The figure shows three views and two pictorial views of one solid part (mm, origin at its lowest corner). Answer the questions. A direction names the side the tool comes from. Round coordinates to 2 decimals unless told otherwise and drop trailing zeros. Order: outer loops, then holes, each group sorted by start corner. A loop starts at its lowest first (then second) coordinate and runs counter-clockwise, first axis right, second up. Notation, with made-up numbers: (-4, 82.25) - (15, 82.25) arc R9 ccw to (15, 92.25) - close; hole circle Ø4 at (32, 39). An arc over 180 degrees is marked (long way). Use CSV: the item, a comma, the result in double quotes.
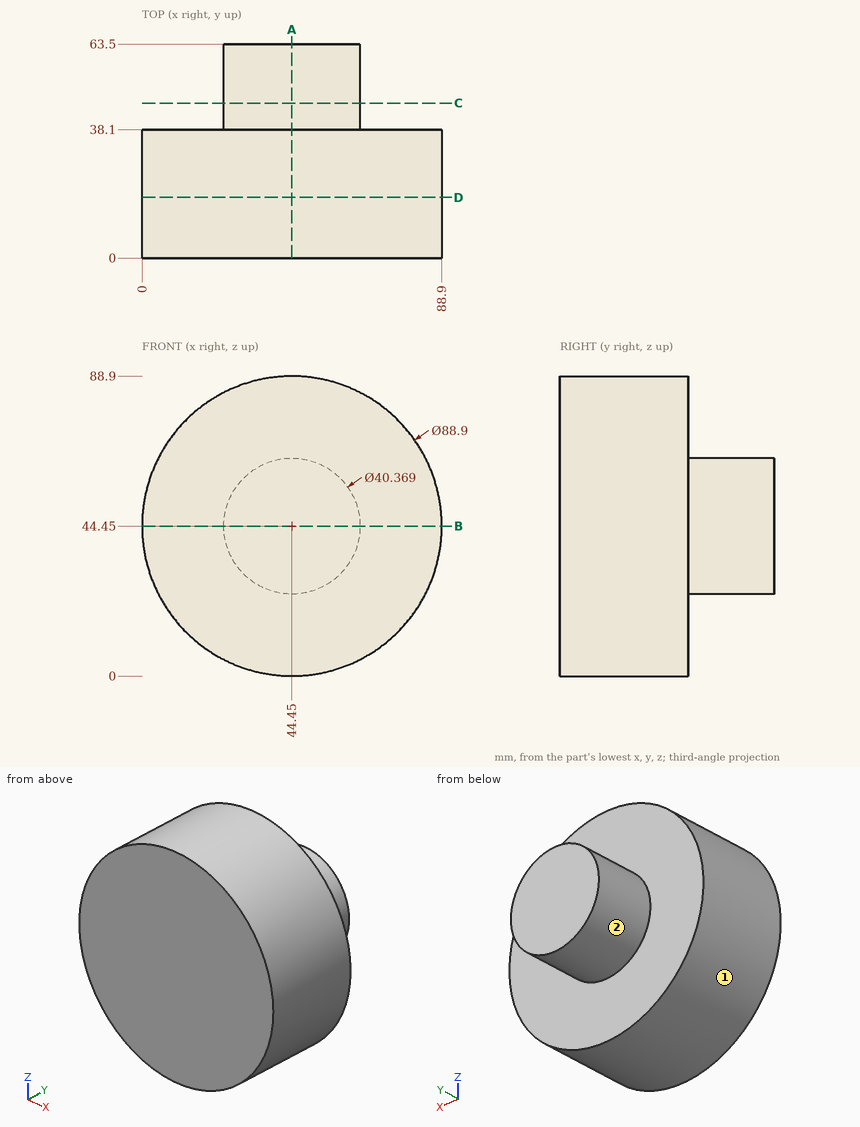
(1) Find section C-C (y = 46). Determine the outline of the cut face in (x, z).
Findings below:
outline,"circle Ø40.37 at (44.45, 44.45)"
(2) Each of these flat-tipped pins is pushed along its axis until it touches: pin 1 (8 mm diameter, centred on x = 70.5, y = 18, fed in from +Z); pin 2 (6 mm diameter, centred on x = 76, z = 49, fed in from +Y); pin 3 (8 mm diameter, centred on y = 10, z = 72, fed in from -X). Where does it stop, or does it pass through?
Findings below:
pin 1,"stops at z = 83.05"
pin 2,"stops at y = 38.1"
pin 3,"stops at x = 6.75"
(3) Find section A-A (x = 44.45). Determine the outline of the cut face in (y, z), and give its area (3 significant figures).
Findings below:
outline,"(0, 0) - (38.1, 0) - (38.1, 24.27) - (63.5, 24.27) - (63.5, 64.63) - (38.1, 64.63) - (38.1, 88.9) - (0, 88.9) - close"
area,"4,410 mm²"
(4) Find section D-D (y = 18). Determine the outline of the cut face in (x, z).
Findings below:
outline,"circle Ø88.9 at (44.45, 44.45)"
(5) Find section B-B (z = 44.45). Determine the outline of the cut face in (x, y).
Findings below:
outline,"(0, 0) - (88.9, 0) - (88.9, 38.1) - (64.63, 38.1) - (64.63, 63.5) - (24.27, 63.5) - (24.27, 38.1) - (0, 38.1) - close"
(6) For the marked faces 1 and 2, determine the directions among +Z, -Z, +X, -X, +Y, -Y from which every point of the face is accessible in a straight line to the end or side of a thin tool.
Findings below:
face 1,"+Y, -Y"
face 2,"+Y"
(7) Find the intervals of material crossed by L1, parallel to Y at x = 18, z = 64.5; L2, parallel to X at y = 52, z = 43.5; L3, parallel to X at y = 38, z = 45, in increasing order. Write a range as from..to.
Findings below:
L1,"y = 0..38.1"
L2,"x = 24.29..64.61"
L3,"x = 0..88.9"
